```python
from build123d import *

# Parameters (mm, degrees)
ESBO_O1_W             = 36
ESBO_O1_H             = 2
FLANGE_BASE2_DEPTH    = 162.5
ESBO_O13_R            = 5
CORTE_EXTRUS_O4_DEPTH = 164.506116094


# Sheet-metal steps are written as plain solids
with BuildPart() as part:
    # Esboço1 → Flange-base2 (new, symmetric)
    with BuildSketch(Plane(origin=(0, 0, 0), x_dir=(0, 0, -1), z_dir=(1, 0, 0))):
        with Locations((0, -1)):
            Rectangle(ESBO_O1_W, ESBO_O1_H)
    extrude(amount=FLANGE_BASE2_DEPTH, both=True)

    # Esboço13 → Corte-extrusão4 (cut, through all)
    with BuildSketch(Plane.XZ.offset(2)):
        with Locations(Location((127.5, 3, 0), (0, 0, 270))):
            Circle(ESBO_O13_R)
    extrude(amount=-CORTE_EXTRUS_O4_DEPTH, mode=Mode.SUBTRACT)


solid = part.part
```
Read the model definition and answer for the solid it produces. Units are mm, in the model's axes. Give positions to 0.01 mm unless a question says otherwise; leave off trailing zeros. Write each loop counter-clockwise with the first axis right and the second up, starting at its lowest first coordinate (ties: lowest second). Pieces come first, ordered by that corner, then holes. Notation, with made-up numbers: (21, -17) -> (43, -17) arc R9 cw to (43, -13) -> close; hole circle Ø3 at (69, 57.5). An arc over 180 degrees is marked (long way). Answer as a JSON object with one key per item and string values.
1) Section A-A on x = 127.5 is taken. Write down the section's boundary in (y, z), then the cut area to 3 significant figures.
Findings below:
{"outline": "(-2, -18) -> (0, -18) -> (0, -2) -> (-2, -2) -> close; (-2, 8) -> (0, 8) -> (0, 18) -> (-2, 18) -> close", "area": "52.0 mm^2"}
2) Straight lines are drawn through the part: probe 1 along X at (y, z) = (-1.15, 3); probe 2 along X at (y, z) = (-1.05, 4). For each, find the intervals that lie inside material, in ascending order. Write a range as from..to.
Findings below:
{"probe 1": "x = -162.5..122.5, 132.5..162.5", "probe 2": "x = -162.5..122.6, 132.4..162.5"}
3) For a pull along Z with two mould halves and no side action, classify faces 1 (the flat face through (2, -2, 0)), 2 (the cylindrical face through (132.457, -1.014, 3.651)) as pulls with the +Z half, pulls with the -Z half, needs draft (parallel to the pull), parting line crosses it, or undercut.
Findings below:
{"face 1": "needs draft", "face 2": "undercut"}
4) Section B-B on z = 3 is taken. Write down the section's boundary in (x, y).
Findings below:
{"outline": "(-162.5, -2) -> (122.5, -2) -> (122.5, 0) -> (-162.5, 0) -> close; (132.5, -2) -> (162.5, -2) -> (162.5, 0) -> (132.5, 0) -> close"}
